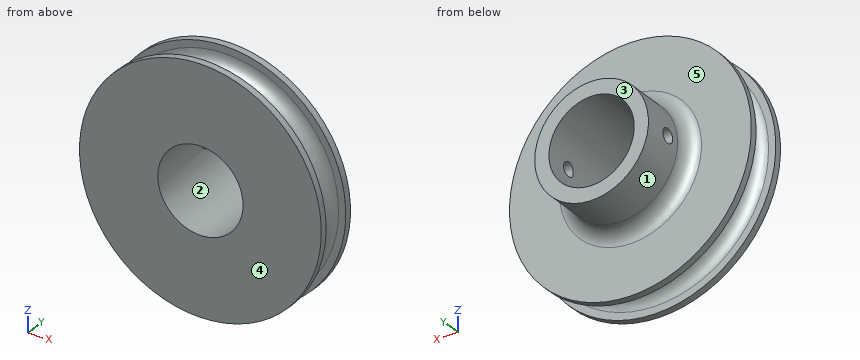
Autodesk Inventor part; units mm, degrees
ref_plane "YZ Plane" through (0, 0, 0) normal (1, 0, 0) x (0, 1, 0)
ref_plane "XZ Plane" through (0, 0, 0) normal (0, 1, 0) x (-1, 0, 0)
ref_plane "XY Plane" through (0, 0, 0) normal (0, 0, 1) x (1, 0, 0)
sketch "Sketch1" plane through (0, 0, 0) normal (1, 0, 0) x (0, 1, 0)
  line L0 (-2.3813, 13.5064) -> (-2.3813, 0) construction
  line L1 (-2.3813, 0) -> (0, 0) construction
  line L2 (2.3813, 0) -> (2.3813, 13.5064)
  line L3 (2.3813, 13.5064) -> (0, 13.5064)
  line L4 (-2.3813, 13.5064) -> (2.3813, 0) construction
  line L5 (-2.3813, 0) -> (2.3813, 13.5064) construction
  line L6 (0, 12.7) -> (0, 11.0871)
  line L7 (0, 11.0871) -> (0, 13.5064)
  line L8 (0, 13.5064) -> (-2.3813, 13.5064) construction
  line L9 (0, 0) -> (2.3813, 0)
  line L10 (0, 11.0871) -> (0, 0)
  arc A0 (0, 11.0871) -> (1.6129, 12.7) centre (0, 12.7) ccw
  line L11 (1.6129, 12.7) -> (1.6129, 13.5064)
  point P0 (0, 6.7532)
  point P1 (0, 6.7532)
  dimension "d2" = 1.6129
  dimension "d4" = 2.3813
  dimension "d5" = 0.8065
  dimension "d16" = 12.7
revolve "Revolution1" add sketch "Sketch1" angle 360 about axis through (0, 0, 0) along (0, 1, 0) contours L9 L10 A0 L11 L3 L2
mirror "Mirror1" about plane through (0, 0, 11.0871) normal (0, -1, 0) of "Revolution1"
sketch "Sketch2" plane through (0, -2.3813, 0) normal (0, -1, 0) x (1, 0, 0)
  circle A0 centre (0, 0) radius 4.7625
  point P0 (0, 0)
  dimension "d7" = 9.525
extrude "Extrusion1" cut sketch "Sketch2" against normal through all
sketch "Sketch3" plane through (0, 2.3813, 0) normal (0, 1, 0) x (1, 0, 0)
  circle A0 centre (0, 0) radius 4.7625
  circle A1 centre (0, 0) radius 6.35
  dimension "d10" = 1.5875
extrude "Extrusion2" add sketch "Sketch3" along normal blind 6.35
sketch "Sketch4" plane through (0, 0, 0) normal (1, 0, 0) x (0, 1, 0)
  circle A0 centre (5.5563, 0) radius 0.7937
  line L0 (8.7312, -6.35) -> (8.7313, 6.35) construction
  line L1 (2.3813, 6.35) -> (2.3812, -6.35) construction
  line L2 (8.7312, -6.35) -> (8.7313, 6.35)
  line L3 (2.3813, 6.35) -> (8.7312, -6.35) construction
  point P0 (0, 0)
  dimension "d13" = 1.5875
extrude "Extrusion3" cut sketch "Sketch4" along normal through all both and the other way through all
fillet "Fillet1" radius 1.5875 1 edges at (-6.35, 2.3813, 0)
equation "\"d5\" = 0.5 * d2"
properties part number "0.5OD_Pulley" material "ABS Plastic"
Source: CAD feature listing. Evaluate the final solid. Frame: model axes, mm. Face numbers are marked on the shaded views. A direction names the side the tool comes from. Round coordinates to 2 decimals unless told otherwise and drop trailing zeros. Loops run counter-clockwise (first coordinate to the right, second up) from the corner with the lowest first, then second, coordinate; pieces in that order, holes last.
1. Contact query for flat-ended pins moving along their axis: pin 1 (4 mm diameter, centred on y = 7, z = 6.5, fed in from +X); pin 2 (4 mm diameter, centred on y = 0, z = 9, fed in from +X); pin 3 (2 mm diameter, centred on y = 5.56, z = 0, fed in from +X). Output: stop coordinate, or through.
2. Ray query, L1, parallel to Y at x = 5.95, z = 0; L2, parallel to Z at x = 0, y = 4.75. Return the intervals inside material, ascending.
3. Section query D-D on y = 3. Output: boundary loops of the cut face in (x, z) (1 decimal).
4. Section query B-B on z = 0. Give the number of separate pieces and of enclosed holes in the cut face, and give its area (3 significant figures).
5. Access query for the marked faces 4 and 5. Directions: +Z, -Z, +X, -X, +Y, -Y. A direction counts if a zero-diameter tool reaches every point of the face in a straight line with its end or side. Return the directions, or none.
6. Mould query, pull axis X, two halves, no side actions, for the marked faces 1, 2 and 3. Classes: released by +X, released by -X, zero draft, split by the parting line, or undercut.
Answers below:
1. pin 1: stops at x = 4.48
1. pin 2: stops at x = 11.01
1. pin 3: stops at x = 6.35
2. L1: y = -2.38 to 4.76, 6.35 to 8.73
2. L2: z = -6.35 to -4.76, 4.76 to 6.35
3. outline: circle Ø13.4 at (0, 0); hole circle Ø9.5 at (0, 0)
4. separate pieces: 4
4. enclosed holes: 0
4. area: 86.1 mm2
5. face 4: +Z, -Z, +X, -X, -Y
5. face 5: +Y
6. face 1: split by the parting line
6. face 2: undercut
6. face 3: zero draft
